from build123d import *

# Parameters (mm, degrees)
SKETCH_R        = 5
SKETCH_R_2      = 3.2
PAD_DEPTH       = 15
SKETCH002_R     = 6.1
POCKET001_DEPTH = 4
SKETCH003_R     = 11.1
POCKET_DEPTH    = 7.4
FILLET_R        = 4
CHAMFER_SIZE    = 0.6
CHAMFER001_SIZE = 0.6
CHAMFER002_SIZE = 0.6


with BuildPart() as part:
    # Sketch → Pad (new body)
    with BuildSketch(Plane.XY):
        Polygon((20, 30), (20, 58), (62.3, 58), (62.3, 30), (82.3, 30), (82.3, 0), (0, 0), (0, 30), align=None)
        with Locations((41.15, 36.85)):
            Circle(SKETCH_R, mode=Mode.SUBTRACT)
        with Locations((11.15, 10)):
            Circle(SKETCH_R_2, mode=Mode.SUBTRACT)
        with Locations((31.15, 10)):
            Circle(SKETCH_R_2, mode=Mode.SUBTRACT)
        with Locations((51.15, 10)):
            Circle(SKETCH_R_2, mode=Mode.SUBTRACT)
        with Locations((71.15, 10)):
            Circle(SKETCH_R_2, mode=Mode.SUBTRACT)
    extrude(amount=PAD_DEPTH)

    # Sketch002 → Pocket001 (cut)
    with BuildSketch(Plane(origin=(0, 0, 0), x_dir=(1, 0, 0), z_dir=(0, 0, -1))):
        with Locations((11.15, -10)):
            Circle(SKETCH002_R)
        with Locations((31.15, -10)):
            Circle(SKETCH002_R)
        with Locations((51.15, -10)):
            Circle(SKETCH002_R)
        with Locations((71.15, -10)):
            Circle(SKETCH002_R)
    extrude(amount=-POCKET001_DEPTH, mode=Mode.SUBTRACT)

    # Sketch003 (on Face5 of Pocket001) → Pocket (cut)
    with BuildSketch(Plane.XY.offset(15)):
        with Locations((41.15, 36.85)):
            Circle(SKETCH003_R)
    extrude(amount=-POCKET_DEPTH, mode=Mode.SUBTRACT)

    # Fillet
    fillet_edges = [part.edges().sort_by_distance(p)[0] for p in [
        (0, 30, 7.5),
        (20, 58, 7.5),
        (62.3, 58, 7.5),
        (82.3, 30, 7.5),
        (82.3, 0, 7.5),
        (0, 0, 7.5),
    ]]
    fillet(fillet_edges, radius=FILLET_R)

    # Chamfer
    chamfer_edges = [part.edges().sort_by_distance(p)[0] for p in [
        (20, 42, 15),
        (21.171573, 56.828427, 15),
        (12, 30, 15),
        (41.15, 58, 15),
        (1.171573, 28.828427, 15),
        (61.128427, 56.828427, 15),
        (0, 15, 15),
        (62.3, 42, 15),
        (1.171573, 1.171573, 15),
        (70.3, 30, 15),
        (41.15, 0, 15),
        (81.128427, 28.828427, 15),
        (81.128427, 1.171573, 15),
        (82.3, 15, 15),
        (47.95, 10, 15),
        (27.95, 10, 15),
        (30.05, 36.85, 15),
        (7.95, 10, 15),
        (67.95, 10, 15),
    ]]
    chamfer(chamfer_edges, length=CHAMFER_SIZE)

    # Chamfer001
    chamfer001_edges = [part.edges().sort_by_distance(p)[0] for p in [
        (20, 42, 0),
        (21.171573, 56.828427, 0),
        (12, 30, 0),
        (41.15, 58, 0),
        (1.171573, 28.828427, 0),
        (61.128427, 56.828427, 0),
        (0, 15, 0),
        (62.3, 42, 0),
        (1.171573, 1.171573, 0),
        (70.3, 30, 0),
        (41.15, 0, 0),
        (81.128427, 28.828427, 0),
        (81.128427, 1.171573, 0),
        (82.3, 15, 0),
        (45.05, 10, 0),
        (25.05, 10, 0),
        (65.05, 10, 0),
        (5.05, 10, 0),
        (36.15, 36.85, 0),
    ]]
    chamfer(chamfer001_edges, length=CHAMFER001_SIZE)

    # Chamfer002
    chamfer002_edges = [part.edges().sort_by_distance(p)[0] for p in [
        (67.95, 10, 4),
        (47.95, 10, 4),
        (27.95, 10, 4),
        (7.95, 10, 4),
    ]]
    chamfer(chamfer002_edges, length=CHAMFER002_SIZE)


solid = part.part
Could you check a few things on this model? Use its own coordinates, in mm. A direction names the side the tool comes from. Round coordinates to 2 decimals unless told otherwise and drop trailing zeros. Order: outer loops, then holes, each group sorted by start corner. A loop starts at its lowest first (then second) coordinate and runs counter-clockwise, first axis right, second up. Notation, with made-up numbers: M -22,51 L -4,51 A18 cw -4,57 Z; hole C 27,14.5 d10. An arc over 180 degrees is marked long. One line per item, written item: value.
(1) Imagine slicing it at A-A (y = 36.85). Write out the boundary of the cut face in (x, z), and give its area (3 significant figures).
Ans:
outline: M 20,0.6 L 20.6,0 L 35.55,0 L 36.15,0.6 L 36.15,7.6 L 30.05,7.6 L 30.05,14.4 L 29.45,15 L 20.6,15 L 20,14.4 Z; M 46.15,0.6 L 46.75,0 L 61.7,0 L 62.3,0.6 L 62.3,14.4 L 61.7,15 L 52.85,15 L 52.25,14.4 L 52.25,7.6 L 46.15,7.6 Z
area: 393 mm^2
(2) Imagine slicing it at C-C (z = 11). Write out the boundary of the cut face in (x, y).
Ans:
outline: M 0,4 A4 ccw 4,0 L 78.3,0 A4 ccw 82.3,4 L 82.3,26 A4 ccw 78.3,30 L 62.3,30 L 62.3,54 A4 ccw 58.3,58 L 24,58 A4 ccw 20,54 L 20,30 L 4,30 A4 ccw 0,26 Z; hole C 11.15,10 d6.4; hole C 31.15,10 d6.4; hole C 41.15,36.85 d22.2; hole C 51.15,10 d6.4; hole C 71.15,10 d6.4
(3) If we mould it in two halves opening along Y, with no side actions, what happens to faces 1 (the conical face through (21.453, 56.491, 0.162)), 2 (the flat face through (8, 13, 4)), 3 (the cylindrical face through (9.828, 15.955, 2.276)), 4 (the flat face through (0, 15, 7))? For each: released by +Y, released by -Y, zero draft, split by the parting line, or undercut.
Ans:
face 1: released by +Y
face 2: undercut
face 3: undercut
face 4: zero draft
(4) I need wall thicknesses on line 1 along X through (y, z) = (10, 7.5); line 2 along X through (y, z) = (11, 9.25); line 3 along Y through (x, z) = (11, 5). Which ranges of each line are inside material? Lowest first, please. Write a range as from..to.
Ans:
line 1: x = 0..7.95, 14.35..27.95, 34.35..47.95, 54.35..67.95, 74.35..82.3
line 2: x = 0..8.11, 14.19..28.11, 34.19..48.11, 54.19..68.11, 74.19..82.3
line 3: y = 0..6.8, 13.2..30
(5) Which directions (+Z, -Z, +X, -X, +Y, -Y) give clear straight access to the entire face, cutting with the end or side of a thin tool? Please do faces 5 (the cylindrical face through (81.097, 28.859, 7.597)), 6 (the cylindrical face through (36.8, 12.3, 2.3)), 7 (the flat face through (20, 42, 7)), 8 (the cylindrical face through (47.12, 46.21, 11.05)), 9 (the flat face through (82.3, 15, 7)).
Ans:
face 5: +Z, -Z, +X, +Y
face 6: -Z
face 7: +Z, -Z, -X, +Y
face 8: +Z
face 9: +Z, -Z, +X, +Y, -Y
(6) Imagine slicing it at D-D (x = 71.15). Write out the boundary of the cut face in (y, z), and give its area (3 significant figures).
Ans:
outline: M 0,0.6 L 0.6,0 L 3.3,0 L 3.9,0.6 L 3.9,4 L 6.2,4 L 6.8,4.6 L 6.8,14.4 L 6.2,15 L 0.6,15 L 0,14.4 Z; M 13.2,4.6 L 13.8,4 L 16.1,4 L 16.1,0.6 L 16.7,0 L 29.4,0 L 30,0.6 L 30,14.4 L 29.4,15 L 13.8,15 L 13.2,14.4 Z
area: 329 mm^2
(7) I'm going to push flat-ended pins straight in: P1, Ø10, axis at x = 50, y = 11, coming from the -Z side; P2, Ø10, axis at x = 51.15, y = 10, coming from the +Z side; P3, Ø6, axis at x = 11.15, y = 10, coming from the -Z side; P4, Ø7.5, axis at x = 31.15, y = 10, coming from the -Z side. Where does each tip first touch, or does it pass through?
Ans:
P1: stops at z = 0.18
P2: stops at z = 15
P3: passes through
P4: stops at z = 4.05
(8) Imagine slicing it at B-B (x = 41.15). Write out the boundary of the cut face in (y, z).
Ans:
outline: M 0,0.6 L 0.6,0 L 31.25,0 L 31.85,0.6 L 31.85,7.6 L 25.75,7.6 L 25.75,14.4 L 25.15,15 L 0.6,15 L 0,14.4 Z; M 41.85,0.6 L 42.45,0 L 57.4,0 L 58,0.6 L 58,14.4 L 57.4,15 L 48.55,15 L 47.95,14.4 L 47.95,7.6 L 41.85,7.6 Z
